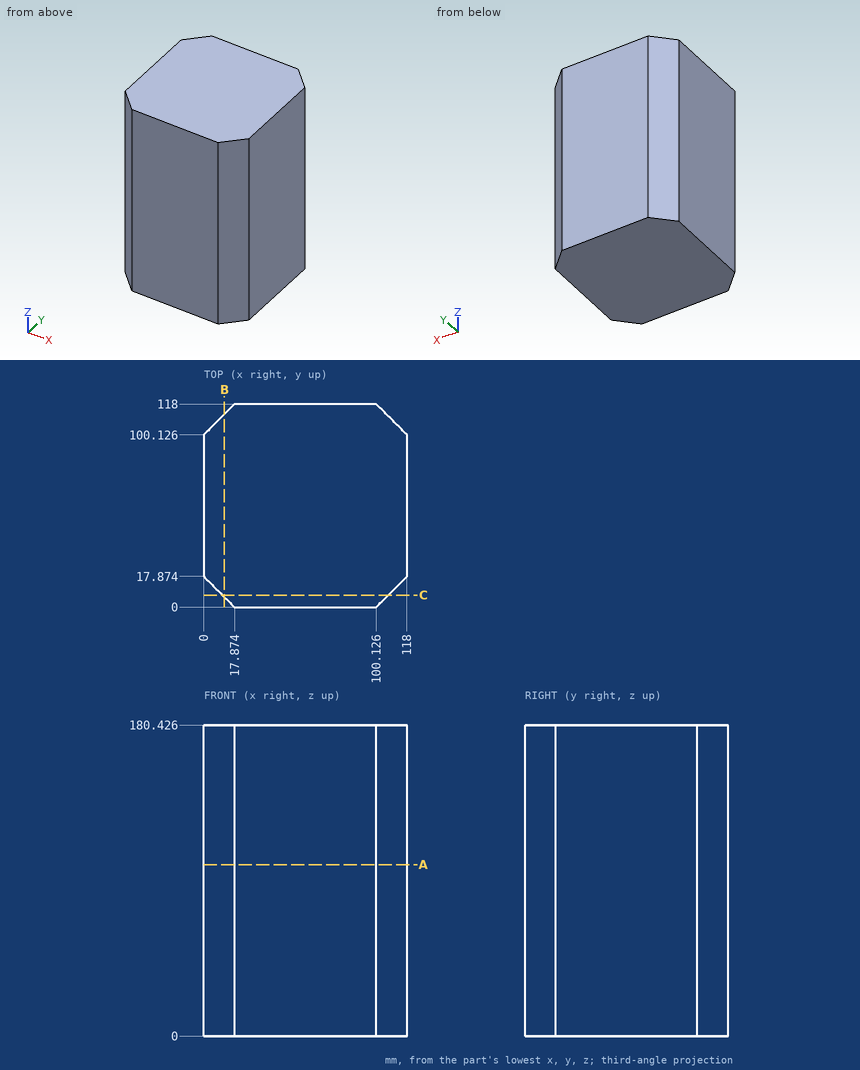
Source: three-view drawing plus pictorial views. Frame: mm from the lowest corner of the part. Give positions to 0.01 mm unless a question says otherwise; leave off trailing zeros. Write each loop counter-clockwise with the first axis right and the second up, starting at its lowest first coordinate (ties: lowest second). Pieces come first, ordered by that corner, then holes. Notation, with made-up numbers: (18, 32) - (32, 32) arc R8 cw to (32, 37) - close; hole circle Ø9 at (64, 58). An arc over 180 degrees is marked (long way). Write item = value, one per line. Start each with the question number.
1. Section query B-B, the plane x = 12. Output: boundary loops of the cut face in (y, z), then the cut area to 3 significant figures.
2. Ray query, L1, parallel to X at y = 16.5, z = 92.5 (1 decimal); L2, parallel to Y at x = 110.5, z = 114 (1 decimal); L3, parallel to Y at x = 103.5, z = 147 (1 decimal). Return the intervals inside material, ascending.
3. Section query A-A, the plane z = 99.5. Output: boundary loops of the cut face in (x, y), then the cut area to 3 significant figures.
4. Section query C-C, the plane y = 7. Output: boundary loops of the cut face in (x, z).
5. First-contact query: pin 1 Ø1.5 at (y, z) = (12, 152) entering from -X. Flat tip, straight axial feed; report the tip coordinate or a pass-through.
Check sheet entries:
q1.outline = (5.87, 0) - (112.13, 0) - (112.13, 180.43) - (5.87, 180.43) - close
q1.area = 19,200 mm2
q2.L1 = 1.4 to 116.6
q2.L2 = 10.4 to 107.6
q2.L3 = 3.4 to 114.6
q3.outline = (0, 17.87) - (17.87, 0) - (100.13, 0) - (118, 17.87) - (118, 100.13) - (100.13, 118) - (17.87, 118) - (0, 100.13) - close
q3.area = 13,300 mm2
q4.outline = (10.87, 0) - (107.13, 0) - (107.13, 180.43) - (10.87, 180.43) - close
q5.pin_1 = 5.12
